Can you work these out from the model? Positions are in its coordinate system, mm. A direction names the side the tool comes from. Coordinates: 2 decimals unless noted, no trailing zeros. Order: outer loops, then holes, each group sorted by start corner. A loop starts at its lowest first (then second) coordinate and runs counter-clockwise, first axis right, second up. Notation, with made-up numbers: (1, -39) -> (13, -39) arc R29 ccw to (13, 0) -> close; hole circle Ø5 at (-37, -17). An arc over 180 degrees is marked (long way). Use a Markdown table: item, result. Add a question column.
1. For faces 1 (the flat face through (-81, 364, 1)), 2 (the flat face through (-30, 364, 7)), 3 (the flat face through (-80, 376, 0)), which set-ups out of +Z, -Z, +X, -X, +Y, -Y let a thin tool reach every point of the face, with its end or its side?
2. Suppose I cut it at D-D, the plane x = -47.5. List the corners of the cut face in (y, z) for me, then the cut area to 3 significant figures.
3. For pin 1 Ø2 at (y, z) = (530, 5) entering from -X; pin 2 Ø4 at (y, z) = (637.5, 3.5) entering from +X; pin 3 Ø4 at (x, z) = (-37, 7) entering from -Y, each with a flat end and sliding along its axis, tell me the tip position at first contact or that it passes through.
4. Suppose I cut it at C-C, the plane z = 5. List the corners of the cut face in (x, y) for me.
5. Suppose I cut it at A-A, the plane x = -86. List the corners of the cut face in (y, z) for me, then the cut area to 3 significant figures.
6. If I drill on line 1 along Z through (x, y) = (-54.5, 41); line 2 along X through (y, z) = (169.5, 6.75); line 3 along Z through (x, y) = (-66, 633.5), over which ranges is the centre line in solid material (lowest first)? Write a range as from..to.
7. Suppose I cut it at B-B, the plane y = 536. List the corners of the cut face in (x, z) for me.
```python
from build123d import *

# Parameters (mm, degrees)
F1_DEPTH = 8
F2_R     = 3
F3_W     = 40
F3_H     = 7
F3_W_2   = 34
F3_W_3   = 25
F4_DEPTH = 1039


with BuildPart() as f1:
    # F0 (on Top) → F1 (new body)
    with BuildSketch(Plane.XY):
        with BuildLine():
            Line((-40, 795), (-95, 795))
            ThreePointArc((-95, 795), (-98.535534, 793.535534), (-100, 790))
            Line((-100, 790), (-100, 771.5))
            Line((-100, 771.5), (-70, 771.5))
            ThreePointArc((-70, 771.5), (-68.93934, 771.06066), (-68.5, 770))
            ThreePointArc((-68.5, 770), (-68.93934, 768.93934), (-70, 768.5))
            Line((-70, 768.5), (-100, 768.5))
            Line((-100, 768.5), (-100, 751.5))
            Line((-100, 751.5), (-70, 751.5))
            ThreePointArc((-70, 751.5), (-68.93934, 751.06066), (-68.5, 750))
            ThreePointArc((-68.5, 750), (-68.93934, 748.93934), (-70, 748.5))
            Line((-70, 748.5), (-100, 748.5))
            Line((-100, 748.5), (-100, 301.5))
            Line((-100, 301.5), (-70, 301.5))
            ThreePointArc((-70, 301.5), (-68.93934, 301.06066), (-68.5, 300))
            ThreePointArc((-68.5, 300), (-68.93934, 298.93934), (-70, 298.5))
            Line((-70, 298.5), (-100, 298.5))
            Line((-100, 298.5), (-100, 281.5))
            Line((-100, 281.5), (-70, 281.5))
            ThreePointArc((-70, 281.5), (-68.93934, 281.06066), (-68.5, 280))
            ThreePointArc((-68.5, 280), (-68.93934, 278.93934), (-70, 278.5))
            Line((-70, 278.5), (-100, 278.5))
            Line((-100, 278.5), (-100, 31.5))
            Line((-100, 31.5), (-70, 31.5))
            ThreePointArc((-70, 31.5), (-68.93934, 31.06066), (-68.5, 30))
            ThreePointArc((-68.5, 30), (-68.93934, 28.93934), (-70, 28.5))
            Line((-70, 28.5), (-100, 28.5))
            Line((-100, 28.5), (-100, 1.5))
            Line((-100, 1.5), (-70, 1.5))
            ThreePointArc((-70, 1.5), (-68.93934, 1.06066), (-68.5, 0))
            ThreePointArc((-68.5, 0), (-68.93934, -1.06066), (-70, -1.5))
            Line((-70, -1.5), (-100, -1.5))
            Line((-100, -1.5), (-100, -50))
            ThreePointArc((-100, -50), (-98.535534, -53.535534), (-95, -55))
            Line((-95, -55), (-40, -55))
            ThreePointArc((-40, -55), (-11.715729, -43.284271), (0, -15))
            Line((0, -15), (0, 755))
            ThreePointArc((0, 755), (-11.715729, 783.284271), (-40, 795))
        make_face()
    extrude(amount=F1_DEPTH)

    # F2
    f2_edges = [f1.edges().sort_by_distance(p)[0] for p in [
        (-100, 771.5, 4),
        (-100, 768.5, 4),
        (-100, 751.5, 4),
        (-100, 748.5, 4),
        (-100, 301.5, 4),
        (-100, 298.5, 4),
        (-100, 281.5, 4),
        (-100, 278.5, 4),
        (-100, 31.5, 4),
        (-100, 28.5, 4),
        (-100, 1.5, 4),
        (-100, -1.5, 4),
    ]]
    fillet(f2_edges, radius=F2_R)

    # F3 (on face) → F4 (cut)
    with BuildSketch(Plane.XZ.offset(55)):
        Polygon((-40, 0), (-40, 7), (-60, 7), (-60, 1), (-60, 0), align=None)
        with Locations((-20, 3.5)):
            Rectangle(F3_W, F3_H)
        with Locations((-78, 4.5)):
            Rectangle(F3_W_2, F3_H)
        with Locations((-107.5, 4.5)):
            Rectangle(F3_W_3, F3_H)
    extrude(amount=-F4_DEPTH, mode=Mode.SUBTRACT)


solid = f1.part
```
Worked out:
| question | item | result |
|---|---|---|
| 1 | face 1 | +Z, -X, +Y, -Y |
| 1 | face 2 | -Z, +X, +Y, -Y |
| 1 | face 3 | -Z, +X, -X, +Y, -Y |
| 2 | outline | (-55, 7) -> (795, 7) -> (795, 8) -> (-55, 8) -> close |
| 2 | area | 850 mm² |
| 3 | pin 1 | stops at x = -61 |
| 3 | pin 2 | stops at x = -60 |
| 3 | pin 3 | stops at y = -54.99 |
| 4 | outline | (-61, -55) -> (-60, -55) -> (-60, 795) -> (-61, 795) -> close |
| 5 | outline | (-55, 0) -> (-1.5, 0) -> (-1.5, 1) -> (-55, 1) -> close; (1.5, 0) -> (28.5, 0) -> (28.5, 1) -> (1.5, 1) -> close; (31.5, 0) -> (278.5, 0) -> (278.5, 1) -> (31.5, 1) -> close; (281.5, 0) -> (298.5, 0) -> (298.5, 1) -> (281.5, 1) -> close; (301.5, 0) -> (748.5, 0) -> (748.5, 1) -> (301.5, 1) -> close; (751.5, 0) -> (768.5, 0) -> (768.5, 1) -> (751.5, 1) -> close; (771.5, 0) -> (795, 0) -> (795, 1) -> (771.5, 1) -> close |
| 5 | area | 832 mm² |
| 6 | line 1 | z = 7..8 |
| 6 | line 2 | x = -61..-60 |
| 6 | line 3 | z = 0..1 |
| 7 | outline | (-100, 0) -> (-60, 0) -> (-60, 7) -> (0, 7) -> (0, 8) -> (-61, 8) -> (-61, 1) -> (-100, 1) -> close |
